from build123d import *

# Parameters (mm, degrees)
F0_R     = 5
F0_W     = 70
F0_H     = 21
F1_DEPTH = 2
F2_W     = 6
F2_H     = 2
F3_DEPTH = 8
F4_R     = 3
F6_DEPTH = 2
F7_W     = 12.8450786794
F7_H     = 2
F8_DEPTH = 13
F9_R     = 3


with BuildPart() as f1:
    # F0 (on Front) → F1 (new body)
    with BuildSketch(Plane.XZ):
        with BuildLine():
            Line((28.9647261798, 43.8778921962), (-51.0352738202, 43.8778921962))
            Line((-51.0352738202, 43.8778921962), (-51.0352738202, -3.1221078038))
            ThreePointArc((-51.0352738202, -3.1221078038), (-50.1565941637, -5.2434281474), (-48.0352738202, -6.1221078038))
            Line((-48.0352738202, -6.1221078038), (-42.0352738202, -6.1221078038))
            Line((-42.0352738202, -6.1221078038), (-42.0352738202, -47.1221078038))
            Line((-42.0352738202, -47.1221078038), (-36.0352738202, -47.1221078038))
            Line((-36.0352738202, -47.1221078038), (-36.0352738202, -40.8721078038))
            Line((-36.0352738202, -40.8721078038), (-16.0352738202, -40.8721078038))
            Line((-16.0352738202, -40.8721078038), (-16.0352738202, -47.1221078038))
            Line((-16.0352738202, -47.1221078038), (-10.0352738202, -47.1221078038))
            Line((-10.0352738202, -47.1221078038), (-10.0352738202, -6.1221078038))
            Line((-10.0352738202, -6.1221078038), (25.9647261798, -6.1221078038))
            ThreePointArc((25.9647261798, -6.1221078038), (28.0860465234, -5.2434281474), (28.9647261798, -3.1221078038))
            Line((28.9647261798, -3.1221078038), (28.9647261798, 43.8778921962))
        make_face()
        with Locations((-26.0352738202, -32.1221078038)):
            Circle(F0_R, mode=Mode.SUBTRACT)
        with Locations((-11.0352738202, 9.3778921962)):
            Rectangle(F0_W, F0_H, mode=Mode.SUBTRACT)
    extrude(amount=F1_DEPTH)

    # F2 (on face) → F3 (join)
    with BuildSketch(Plane.XZ.offset(2)):
        with Locations((-39.0352738202, -46.1221078038)):
            Rectangle(F2_W, F2_H)
        with Locations((-13.0352738202, -46.1221078038)):
            Rectangle(F2_W, F2_H)
    extrude(amount=F3_DEPTH)

    # F4
    f4_edges = [f1.edges().sort_by_distance(p)[0] for p in [
        (-13.035274, 0, -47.122108),
        (-39.035274, 0, -47.122108),
    ]]
    fillet(f4_edges, radius=F4_R)

    # F5 (on face) → F6 (join)
    with BuildSketch(Plane.XY.offset(43.8778921962)):
        Polygon((-51.0352738202, 8), (-51.0352738202, 0), (28.9647261798, 0), (28.9647261798, 8), (-11.7104330932, 38), (-11.7104330932, 58), (-24.5555117726, 58), (-24.5555117726, 38), align=None)
    extrude(amount=-F6_DEPTH)

    # F7 (on face) → F8 (join)
    with BuildSketch(Plane(origin=(0, 0, 41.8778921962), x_dir=(1, 0, 0), z_dir=(0, 0, -1))):
        with Locations((-18.1329724329, -57)):
            Rectangle(F7_W, F7_H)
    extrude(amount=F8_DEPTH)

    # F9
    f9_edges = [f1.edges().sort_by_distance(p)[0] for p in [
        (-18.132972, 58, 43.877892),
        (-11.035274, -2, 43.877892),
    ]]
    fillet(f9_edges, radius=F9_R)


solid = f1.part
Read the model definition and answer for the solid it produces. Units are mm, in the model's axes. A direction names the side the tool comes from. Give positions to 0.01 mm unless a question says otherwise; leave off trailing zeros. Loops run counter-clockwise (first coordinate to the right, second up) from the corner with the lowest first, then second, coordinate; pieces in that order, holes last. Notation, with made-up numbers: (64, -32) - (72, -32) arc R19 cw to (72, 4) - close; hole circle Ø6 at (8, -14). An arc over 180 degrees is marked (long way). Answer as CSV lines item,"result". Start each with the question number.
1) Find section D-D (x = -27.5). Write down the section's boundary in (y, z).
2) Find section A-A (z = 7.5). Write down the section's boundary in (x, y).
3) Find section C-C (z = 30). Write down the section's boundary in (x, y).
4) Straight lines are drawn through the part: L1, parallel to Y at x = -34, z = 35.5; L2, parallel to Z at x = -9.5, y = 32.5. For each, find the intervals that lie inside material, in ascending order. Write a range as from..to.
5) Find section B-B (x = -6.5). Write down the section's boundary in (y, z), then the cut area to 3 significant figures.
6) Determine the mould class of faces 1 (the face through (-38.993, -0.902, -46.267)), 2 (the face through (28.06, -0.99, -5.27)), 3 (the face through (-18, 56, 35)) for opening direction Y: released by +Y, released by -Y, zero draft, split by the parting line, or undercut.
7) Which of the six approach directions +Z, -Z, +X, -X, +Y, -Y give full straight-line access (tool end or side, diameter ignored) to faces 4 (the face through (-11.71, 52, 43)), 5 (the face through (-36.035, -3.8, -45.4)), 6 (the face through (-13, -6, -45.122))?
8) Each of these flat-tipped pins is pushed along its axis until it touches: pin 1 Ø8 at (x, z) = (18.5, 9) entering from -Y (3 decimals); pin 2 Ø10.5 at (x, z) = (-15, 36) entering from -Y; pin 3 Ø10 at (x, y) = (-24, 10.5) entering from -Z; pin 4 Ø1.6 at (x, y) = (-16.5, 57) entering from -Z. Where does it stop, or does it pass through?
Findings below:
1,outline,"(-2, -40.87) - (0, -40.87) - (0, -36.9) - (-2, -36.9) - close; (-2, -27.34) - (0, -27.34) - (0, -1.12) - (-2, -1.12) - close; (-2, 19.88) - (0, 19.88) - (0, 41.88) - (34.66, 41.88) - (34.66, 43.88) - (1, 43.88) arc R3 ccw to (-2, 40.88) - close"
2,outline,"(-51.04, -2) - (-46.04, -2) - (-46.04, 0) - (-51.04, 0) - close; (23.96, -2) - (28.96, -2) - (28.96, 0) - (23.96, 0) - close"
3,outline,"(-51.04, -2) - (28.96, -2) - (28.96, 0) - (-51.04, 0) - close; (-24.56, 56) - (-11.71, 56) - (-11.71, 58) - (-24.56, 58) - close"
4,L1,"-2..0"
4,L2,"41.88..43.88"
5,outline,"(-2, -6.12) - (0, -6.12) - (0, -1.12) - (-2, -1.12) - close; (-2, 19.88) - (0, 19.88) - (0, 41.88) - (34.16, 41.88) - (34.16, 43.88) - (1, 43.88) arc R3 ccw to (-2, 40.88) - close"
5,area,"124 mm^2"
6,face 1,"released by +Y"
6,face 2,"zero draft"
6,face 3,"undercut"
7,face 4,"+Z, -Z, +X, +Y"
7,face 5,"-Z, +Y, -Y"
7,face 6,"+Z, +X, -X, -Y"
8,pin 1,"through"
8,pin 2,"y = -2"
8,pin 3,"z = 41.88"
8,pin 4,"z = 28.88"
